Design review of the part built by this model. Coordinates are the model's own, in mm. A direction names the side the tool comes from. Give positions to 0.01 mm unless a question says otherwise; leave off trailing zeros. Write each loop counter-clockwise with the first axis right and the second up, starting at its lowest first coordinate (ties: lowest second). Pieces come first, ordered by that corner, then holes. Notation, with made-up numbers: (61, -12.75) -> (82, -12.75) arc R25 cw to (82, 4.25) -> close; hole circle Ø6 at (-14.5, 89). An arc over 180 degrees is marked (long way). Return JSON: item names as keys, results as strings. Group by question number.
from build123d import *

# Parameters (mm, degrees)
F1_DEPTH       = 12.7
F3_D           = 3.3
F3_CBORE_D     = 6.5
F3_CBORE_DEPTH = 0
F4_R           = 2.54


with BuildPart() as f1:
    # F0 (on Front) → F1 (new body)
    with BuildSketch(Plane.XZ):
        with BuildLine():
            ThreePointArc((0, 12.7), (-6.35, 6.35), (0, 0))
            Line((0, 0), (25.4, 0))
            Line((25.4, 0), (25.4, 6.35))
            Line((25.4, 6.35), (76.2, 6.35))
            Line((76.2, 6.35), (76.2, 12.7))
            Line((76.2, 12.7), (19.05, 12.7))
            Line((19.05, 12.7), (0, 12.7))
        make_face()
    extrude(amount=F1_DEPTH)

    # F3 (through all)
    with Locations(Plane.XZ.offset(12.7)):
        with Locations((0, 6.35)):
            CounterBoreHole(F3_D / 2, F3_CBORE_D / 2, F3_CBORE_DEPTH)

    # F4
    f4_edges = [f1.edges().sort_by_distance(p)[0] for p in [
        (76.2, -12.7, 9.525),
        (76.2, -6.35, 6.35),
        (76.2, -6.35, 12.7),
        (76.2, 0, 9.525),
    ]]
    fillet(f4_edges, radius=F4_R)


solid = f1.part
Q1. Mouldability with a two-part tool opening along Z and no side actions: class faces 1 (the face through (0.36, -6.26, 4.74)), 2 (the face through (13, -6, 0)), 3 (the face through (25.4, -6, 3)) as +Z half, -Z half, draft (parallel to the pull), parting line (faces both ways), or undercut.
Q2. For L1, parallel to Z at x = 0, y = -2.75; L2, parallel to X at y = -7.75, z = 6.25; L3, parallel to Z at x = 59, y = -3, list the stretches that pass through material, from the lowest coordinate up. Write a range as from..to.
Q3. Tool access review of faces 4 (the face through (24, -12.7, 8)), 5 (the face through (49, -6, 6.35)): name each direction out of +Z, -Z, +X, -X, +Y, -Y from which nothing blocks a thin tool from reaching the whole face with its end or side.
Q4. Take a section at B-B, the plane x = 40. Give the boundary of the cut face in (y, z).
Q5. Take a section at A-A, the plane y = -8. Give the boundary of the cut face in (x, z).
Q6. Insertion check: pin 1 (7 mm diameter, centred on y = -8, z = 4, fed in from +X); pin 2 (6 mm diameter, centred on y = -5.5, z = 3, fed in from -X); pin 3 (1.5 mm diameter, centred on y = -2.5, z = 5.5, fed in from +X). Each pin has a flat end and moves straight along its axis. Give the tip position at first contact, or say it passes through.
Final values:
{
 "1": {"face 1": "undercut", "face 2": "-Z half", "face 3": "draft"},
 "2": {"L1": "z = 0..4.7, 8..12.7", "L2": "x = -6.35..-1.65, 1.65..25.4", "L3": "z = 6.35..12.7"},
 "3": {"face 4": "+Z, -Z, +X, -X, -Y", "face 5": "-Z, +X, +Y, -Y"},
 "4": {"outline": "(-12.7, 6.35) -> (0, 6.35) -> (0, 12.7) -> (-12.7, 12.7) -> close"},
 "5": {"outline": "(0, 0) -> (25.4, 0) -> (25.4, 6.35) -> (73.66, 6.35) arc R2.54 ccw to (76.2, 8.89) -> (76.2, 10.16) arc R2.54 ccw to (73.66, 12.7) -> (0, 12.7) arc R6.35 ccw to start; hole circle Ø3.3 at (0, 6.35)"},
 "6": {"pin 1": "stops at x = 75.79", "pin 2": "stops at x = -6.34", "pin 3": "stops at x = 25.4"}
}
